```python
from build123d import *

# Parameters (mm, degrees)
SKETCH1_W                               = 94.087856827
SKETCH1_H                               = 63.5
SKETCH1_R                               = 25
BOSS_EXTRUDE1_DEPTH                     = 46.387125
CBORE_FOR_M5_HEX_HEAD_BOLT1_D           = 5.5
CBORE_FOR_M5_HEX_HEAD_BOLT1_CBORE_D     = 12.24
CBORE_FOR_M5_HEX_HEAD_BOLT1_CBORE_DEPTH = 10
CBORE_FOR_M5_HEX_HEAD_BOLT2_D           = 5.5
CBORE_FOR_M5_HEX_HEAD_BOLT2_CBORE_D     = 12.24
CBORE_FOR_M5_HEX_HEAD_BOLT2_CBORE_DEPTH = 10
HOLE_FOR_6_300_SC_NUTS_SP_1_D           = 4.7625
HOLE_FOR_6_300_SC_NUTS_SP_1_DEPTH       = 12.7
HOLE_FOR_6_300_SC_NUTS_SP_1_TIP         = 1.430799349


with BuildPart() as part:
    # Sketch1 → Boss-Extrude1 (new body)
    with BuildSketch(Plane.ZY.offset(-20.770136657)):
        with Locations((248.31612335, 301.367904211)):
            Rectangle(SKETCH1_W, SKETCH1_H)
        with Locations((236.197194936, 301.367904211)):
            Circle(SKETCH1_R, mode=Mode.SUBTRACT)
    extrude(amount=BOSS_EXTRUDE1_DEPTH)

    # CBORE for M5 Hex Head Bolt1 (through all)
    with Locations(Plane(origin=(20.770136657, 0, 0), x_dir=(0, 0, -1), z_dir=(1, 0, 0))):
        with Locations((-259.178165324, 324.348874599), (-259.178165324, 278.386933822), (-213.216224547, 278.386933822), (-213.216224547, 324.348874599)):
            CounterBoreHole(CBORE_FOR_M5_HEX_HEAD_BOLT1_D / 2, CBORE_FOR_M5_HEX_HEAD_BOLT1_CBORE_D / 2, CBORE_FOR_M5_HEX_HEAD_BOLT1_CBORE_DEPTH)

    # CBORE for M5 Hex Head Bolt2 (through all)
    with Locations(Plane.ZY.offset(25.616988343)):
        with Locations((282.660051763, 314.067904211), (282.660051763, 288.667904211)):
            CounterBoreHole(CBORE_FOR_M5_HEX_HEAD_BOLT2_D / 2, CBORE_FOR_M5_HEX_HEAD_BOLT2_CBORE_D / 2, CBORE_FOR_M5_HEX_HEAD_BOLT2_CBORE_DEPTH)

    # Hole for #6 300® SC Nuts (SP)1
    with Locations(Plane(origin=(20.770136657, 0, 0), x_dir=(0, 0, -1), z_dir=(1, 0, 0))):
        with Locations((-206.034694936, 301.367904211)):
            Hole(HOLE_FOR_6_300_SC_NUTS_SP_1_D / 2, depth=HOLE_FOR_6_300_SC_NUTS_SP_1_DEPTH)
            with Locations((0, 0, -(HOLE_FOR_6_300_SC_NUTS_SP_1_DEPTH + HOLE_FOR_6_300_SC_NUTS_SP_1_TIP / 2))):  # 118° drill point
                Cone(0, HOLE_FOR_6_300_SC_NUTS_SP_1_D / 2, HOLE_FOR_6_300_SC_NUTS_SP_1_TIP, mode=Mode.SUBTRACT)


solid = part.part
```
Here's how the part is built. I have some questions about the finished solid (model axes, mm). A direction names the side the tool comes from. Round coordinates to 2 decimals unless told otherwise and drop trailing zeros. Loops run counter-clockwise (first coordinate to the right, second up) from the corner with the lowest first, then second, coordinate; pieces in that order, holes last.
1. Thinking about a two-plate mould opening in Y: for faces 1 (the face through (-2, 269.618, 248)), 2 (the face through (-25.617, 316, 258)), 3 (the face through (15.84, 272.41, 260.5)), which applies, released by +Y, released by -Y, zero draft, split by the parting line, or undercut?
Answers:
face 1: released by -Y
face 2: zero draft
face 3: undercut
2. If I drill on probe 1 along Y at (x, z) = (1.5, 221.5); probe 2 along Z at (x, y) = (-19.5, 285); probe 3 along Y at (x, z) = (-23, 214.5), over which ranges is the centre line in solid material (lowest first)?
Answers:
probe 1: y = 269.62 to 281.14, 321.59 to 333.12
probe 2: z = 201.27 to 217.3, 255.09 to 277.76, 287.56 to 295.36
probe 3: y = 269.62 to 275.95, 280.82 to 288.95, 313.79 to 321.92, 326.78 to 333.12
3. Suppose I cut it at C-C, the plane z = 214. Please give me the cut outline in (x, y), and give its area (3 significant figures).
Answers:
outline: (-25.62, 269.62) - (20.77, 269.62) - (20.77, 272.32) - (10.77, 272.32) - (10.77, 275.75) - (-25.62, 275.75) - close; (-25.62, 281.02) - (10.77, 281.02) - (10.77, 284.46) - (20.77, 284.46) - (20.77, 289.87) - (-25.62, 289.87) - close; (-25.62, 312.87) - (20.77, 312.87) - (20.77, 318.28) - (10.77, 318.28) - (10.77, 321.71) - (-25.62, 321.71) - close; (-25.62, 326.98) - (10.77, 326.98) - (10.77, 330.42) - (20.77, 330.42) - (20.77, 333.12) - (-25.62, 333.12) - close
area: 1,250 mm2
4. Suppose I cut it at B-B, the plane y = 323. Please give me the cut outline in (x, z).
Answers:
outline: (-25.62, 201.27) - (20.77, 201.27) - (20.77, 207.25) - (10.77, 207.25) - (10.77, 210.82) - (-25.62, 210.82) - close; (-25.62, 215.61) - (10.77, 215.61) - (10.77, 219.19) - (20.77, 219.19) - (20.77, 223.67) - (-25.62, 223.67) - close; (-25.62, 248.73) - (20.77, 248.73) - (20.77, 253.21) - (10.77, 253.21) - (10.77, 256.78) - (-25.62, 256.78) - close; (-25.62, 261.57) - (10.77, 261.57) - (10.77, 265.15) - (20.77, 265.15) - (20.77, 295.36) - (-25.62, 295.36) - close
5. For faces 4 (the face through (-20.687, 310.344, 277.803)), 5 (the face through (15.84, 272.41, 214.54)), 6 (the face through (2.831, 290.526, 284.687)), which set-ups out of +Z, -Z, +X, -X, +Y, -Y let a thin tool reach every point of the face, with its end or its side?
Answers:
face 4: -X
face 5: +X
face 6: +X, -X
6. Suppose I cut it at D-D, the plane x = 15. Give the number of separate pieces and of enclosed holes in the cut face, and give its area (3 significant figures).
Answers:
separate pieces: 1
enclosed holes: 8
area: 3,480 mm2
7. Suppose I cut it at A-A, the plane z = 228. Please give me the cut outline in (x, y), and give its area (3 significant figures).
Answers:
outline: (-25.62, 269.62) - (20.77, 269.62) - (20.77, 277.75) - (-25.62, 277.75) - close; (-25.62, 324.99) - (20.77, 324.99) - (20.77, 333.12) - (-25.62, 333.12) - close
area: 754 mm2
8. Will these pins go through, and if not, where does the flat tip stop? pin 1 (3.5 mm diameter, centred on y = 327, z = 213, fed in from +X); pin 2 (6 mm diameter, centred on y = 313.5, z = 285, fed in from -X); pin 3 (3.5 mm diameter, centred on y = 324.35, z = 259.18, fed in from +X).
Answers:
pin 1: stops at x = 10.77
pin 2: stops at x = -15.62
pin 3: passes through
